```python
from build123d import *

# Parameters (mm, degrees)
SKETCH2_R               = 1.5875
BOSS_EXTRUDE1_DEPTH     = 10
BOSS_EXTRUDE2_DEPTH     = 120
SKETCH4_R               = 4.0875
CUT_EXTRUDE1_DEPTH      = 30.5
CUT_EXTRUDE1_DEPTH_BACK = 30.5
SKETCH5_R               = 4.0875
CUT_EXTRUDE2_DEPTH      = 31
SKETCH6_R               = 4.0875
CUT_EXTRUDE3_DEPTH      = 31
FILLET1_R               = 10
SKETCH7_R               = 1.75
CUT_EXTRUDE4_DEPTH      = 4
CUT_EXTRUDE5_DEPTH      = 2.25


with BuildPart() as part:
    # Sketch2 → Boss-Extrude1 (new body)
    with BuildSketch(Plane.XY):
        with BuildLine():
            Line((0, -27.7495), (0, 0))
            Line((0, 0), (38.1, 0))
            ThreePointArc((38.1, 0), (-26.940768363, 26.940768363), (0, -38.1))
            Line((0, -38.1), (0, -30.9245))
            ThreePointArc((0, -30.9245), (-1.5875, -29.337), (0, -27.7495))
        make_face()
        with Locations((-25.406587271, 14.6685)):
            Circle(SKETCH2_R, mode=Mode.SUBTRACT)
        with Locations((25.406587271, 14.6685)):
            Circle(SKETCH2_R, mode=Mode.SUBTRACT)
        with BuildLine():
            Line((38.1, 0), (0, 0))
            Line((0, 0), (0, -27.7495))
            ThreePointArc((0, -27.7495), (1.122532015, -28.214467985), (1.5875, -29.337))
            ThreePointArc((1.5875, -29.337), (1.122532015, -30.459532015), (0, -30.9245))
            Line((0, -30.9245), (0, -38.1))
            ThreePointArc((0, -38.1), (26.940768363, -26.940768363), (38.1, 0))
        make_face()
    extrude(amount=BOSS_EXTRUDE1_DEPTH)


with BuildPart() as body_2:
    # Sketch3 → Boss-Extrude2 (new body)
    with BuildSketch(Plane.XY.offset(10)):
        with BuildLine():
            ThreePointArc((29.494087271, 14.6685), (24.324372064, 18.610132466), (21.892146477, 12.581309985))
            Line((21.892146477, 12.581309985), (23.37551462, 15.150578976))
            ThreePointArc((23.37551462, 15.150578976), (25.649272347, 16.741845172), (27.494087271, 14.6685))
            ThreePointArc((27.494087271, 14.6685), (27.323499399, 13.841998855), (26.839616236, 13.150578976))
            Line((26.839616236, 13.150578976), (25.356248092, 10.581309985))
            ThreePointArc((25.356248092, 10.581309985), (28.279033516, 11.760457906), (29.494087271, 14.6685))
        make_face()
        with BuildLine():
            Line((24.362837271, 12.86067197), (23.362837271, 11.128621162))
            ThreePointArc((23.362837271, 11.128621162), (24.324372064, 10.726867534), (25.356248092, 10.581309985))
            Line((25.356248092, 10.581309985), (26.839616236, 13.150578976))
            ThreePointArc((26.839616236, 13.150578976), (25.649272347, 12.595154828), (24.362837271, 12.86067197))
        make_face()
        with BuildLine():
            ThreePointArc((21.892146477, 12.581309985), (22.534141026, 11.760457906), (23.362837271, 11.128621162))
            Line((23.362837271, 11.128621162), (24.362837271, 12.86067197))
            ThreePointArc((24.362837271, 12.86067197), (23.489675143, 13.841998855), (23.37551462, 15.150578976))
            Line((23.37551462, 15.150578976), (21.892146477, 12.581309985))
        make_face()
        with BuildLine():
            Line((23.362837271, 11.128621162), (2.04375, -25.797121162))
            ThreePointArc((2.04375, -25.797121162), (2.872446245, -26.428957906), (3.514440794, -27.249809985))
            Line((3.514440794, -27.249809985), (25.356248092, 10.581309985))
            ThreePointArc((25.356248092, 10.581309985), (24.324372064, 10.726867534), (23.362837271, 11.128621162))
        make_face()
        with BuildLine():
            ThreePointArc((0.050339179, -25.249809985), (1.082215206, -25.395367534), (2.04375, -25.797121162))
            Line((2.04375, -25.797121162), (23.362837271, 11.128621162))
            ThreePointArc((23.362837271, 11.128621162), (22.534141026, 11.760457906), (21.892146477, 12.581309985))
            Line((21.892146477, 12.581309985), (0.050339179, -25.249809985))
        make_face()
        with BuildLine():
            ThreePointArc((-1.433028965, -27.819078976), (-0.242685076, -27.263654828), (1.04375, -27.52917197))
            Line((1.04375, -27.52917197), (2.04375, -25.797121162))
            ThreePointArc((2.04375, -25.797121162), (1.082215206, -25.395367534), (0.050339179, -25.249809985))
            Line((0.050339179, -25.249809985), (-1.433028965, -27.819078976))
        make_face()
        with BuildLine():
            Line((2.04375, -25.797121162), (1.04375, -27.52917197))
            ThreePointArc((1.04375, -27.52917197), (1.80782803, -28.29325), (2.0875, -29.337))
            ThreePointArc((2.0875, -29.337), (2.073345172, -29.579685076), (2.03107265, -29.819078976))
            Line((2.03107265, -29.819078976), (3.514440794, -27.249809985))
            ThreePointArc((3.514440794, -27.249809985), (2.872446245, -26.428957906), (2.04375, -25.797121162))
        make_face()
        with BuildLine():
            ThreePointArc((2.03107265, -29.819078976), (-1.04375, -31.14482803), (-1.433028965, -27.819078976))
            Line((-1.433028965, -27.819078976), (0.050339179, -25.249809985))
            ThreePointArc((0.050339179, -25.249809985), (-2.908042094, -32.209446245), (4.0875, -29.337))
            ThreePointArc((4.0875, -29.337), (3.941632466, -28.254784794), (3.514440794, -27.249809985))
            Line((3.514440794, -27.249809985), (2.03107265, -29.819078976))
        make_face()
    extrude(amount=BOSS_EXTRUDE2_DEPTH)

    # Sketch4 → Cut-Extrude1 (cut, two sides)
    with BuildSketch(Plane.XY.offset(70)) as cut_extrude1_sk:
        with Locations((0, -29.337)):
            Circle(SKETCH4_R)
    extrude(amount=CUT_EXTRUDE1_DEPTH, mode=Mode.SUBTRACT)
    extrude(cut_extrude1_sk.sketch, amount=-CUT_EXTRUDE1_DEPTH_BACK, mode=Mode.SUBTRACT)

    # Sketch5 → Cut-Extrude2 (cut)
    with BuildSketch(Plane(origin=(0, 0, 10), x_dir=(-1, 0, 0), z_dir=(0, 0, -1))):
        with Locations((-25.406587271, 14.6685)):
            Circle(SKETCH5_R)
    extrude(amount=-CUT_EXTRUDE2_DEPTH, mode=Mode.SUBTRACT)

    # Sketch6 → Cut-Extrude3 (cut)
    with BuildSketch(Plane.XY.offset(130)):
        with Locations((25.406587271, 14.6685)):
            Circle(SKETCH6_R)
    extrude(amount=-CUT_EXTRUDE3_DEPTH, mode=Mode.SUBTRACT)

    # Fillet1
    fillet1_edges = [body_2.edges().sort_by_distance(p)[0] for p in [
        (0.050339179, -25.249809985, 115.25),
        (3.514440794, -27.249809985, 115.25),
        (0.050339179, -25.249809985, 24.75),
        (3.514440794, -27.249809985, 24.75),
        (21.892146477, 12.581309985, 70),
        (25.356248092, 10.581309985, 70),
    ]]
    fillet(fillet1_edges, radius=FILLET1_R)

    # Sketch7 → Cut-Extrude4 (cut)
    with BuildSketch(Plane(origin=(10.971242828, -6.33425, 0), x_dir=(0, 0, 1), z_dir=(-0.866025404, 0.5, 0))):
        with Locations((23.771980031, -8.948916416)):
            Circle(SKETCH7_R)
        with Locations((23.771980031, 16.095483584)):
            Circle(SKETCH7_R)
        with Locations((118.488580031, 16.095483584)):
            Circle(SKETCH7_R)
        with Locations((118.488580031, -8.948916416)):
            Circle(SKETCH7_R)
    extrude(amount=-CUT_EXTRUDE4_DEPTH, mode=Mode.SUBTRACT)

    # Sketch8 → Cut-Extrude5 (cut)
    with BuildSketch(Plane(origin=(14.435344443, -8.33425, 0), x_dir=(0, 0, -1), z_dir=(0.866025404, -0.5, 0))):
        Polygon((-19.812511885, 16.095483584), (-21.792245958, 19.524483584), (-25.751714104, 19.524483584), (-27.731448177, 16.095483584), (-25.751714104, 12.666483584), (-21.792245958, 12.666483584), align=None)
        Polygon((-19.812511885, -8.948916416), (-21.792245958, -5.519916416), (-25.751714104, -5.519916416), (-27.731448177, -8.948916416), (-25.751714104, -12.377916416), (-21.792245958, -12.377916416), align=None)
        Polygon((-114.529111885, 16.095483584), (-116.508845958, 19.524483584), (-120.468314104, 19.524483584), (-122.448048177, 16.095483584), (-120.468314104, 12.666483584), (-116.508845958, 12.666483584), align=None)
        Polygon((-114.529111885, -8.948916416), (-116.508845958, -5.519916416), (-120.468314104, -5.519916416), (-122.448048177, -8.948916416), (-120.468314104, -12.377916416), (-116.508845958, -12.377916416), align=None)
    extrude(amount=-CUT_EXTRUDE5_DEPTH, mode=Mode.SUBTRACT)


solid = body_2.part
```
Verification items for the finished model (mm, model axes). A direction names the side the tool comes from. Coordinates: 2 decimals unless noted, no trailing zeros. Loops run counter-clockwise (first coordinate to the right, second up) from the corner with the lowest first, then second, coordinate; pieces in that order, holes last. Notation, with made-up numbers: (-21, 67) -> (8, 67) arc R12 ccw to (8, 87) -> close; hole circle Ø4 at (88.5, -11.5). An arc over 180 degrees is marked (long way). Answer in a Markdown table with one row per item. Add a question column.
1. Section check B-B, the plane y = -7. Enter the section's corners in (x, z).
2. Depth check by flat-ended pin: P1, Ø6, axis at y = -22, z = 59.5, coming from the -X side; P2, Ø12, axis at y = -8, z = 98.5, coming from the +X side; P3, Ø10, axis at x = 15.5, z = 95.5, coming from the -Y side. Enter the tip coordinate at first touch or a pass-through.
3. Material ranges on probe 1 along Y at (x, z) = (0, 115); probe 2 along X at (y, z) = (-8, 110); probe 3 along X at (y, z) = (-16, 34), recorded low to high. Write a range as [from, to].
4. Section check A-A, the plane z = 60. Enter the section's corners in (x, y) (1 decimal).
5. Draft check along Y on faces 1 (the face through (22.392, 7.665, 121.444)), 2 (the face through (27, 13, 41)), 3 (the face through (8.417, -14.258, 120.304)), 4 (the face through (0.297, -24.088, 24.956)). Enter one of: +Y half, -Y half, draft (parallel to the pull), parting line (faces both ways), or undercut.
6. Access from +Z, -Z, +X, -X, +Y, -Y to the whole of each face (thin tool, end or side, straight path). Record for faces 5 (the face through (20.94, 7.43, 25.59)), 6 (the face through (23.388, 11.114, 25.283)), 7 (the face through (23.34, 11.14, 114.72)), 8 (the face through (11, -12, 10)).
Derived:
| question | item | result |
|---|---|---|
| 1 | outline | (10.59, 10) -> (15.21, 10) -> (15.21, 130) -> (10.59, 130) -> close |
| 2 | P1 | stops at x = 0.19 |
| 2 | P2 | stops at x = 18.09 |
| 2 | P3 | stops at y = -15.15 |
| 3 | probe 1 | y = [-33.42, -31.42], [-27.25, -24.37] |
| 3 | probe 2 | x = [10.01, 14.63] |
| 3 | probe 3 | x = [5.39, 10.01] |
| 4 | outline | (0.1, -25.2) arc R4.1 cw to (3.5, -27.2) -> (23.4, 7.3) arc R10 cw to (27.4, 11.1) arc R4.1 ccw (long way) to (21.3, 14.6) arc R10 cw to (20, 9.3) -> close; hole circle Ø4.2 at (25.4, 14.7) |
| 5 | face 1 | undercut |
| 5 | face 2 | draft |
| 5 | face 3 | undercut |
| 5 | face 4 | +Y half |
| 6 | face 5 | none |
| 6 | face 6 | -Z, +X, +Y |
| 6 | face 7 | +Z, +X, +Y |
| 6 | face 8 | -Z, +X, -X, +Y, -Y |
